Check sheet for the modelled part. Datum: model origin and axes. Units: mm. A direction names the side the tool comes from. Coordinates: 2 decimals unless noted, no trailing zeros. Loops run counter-clockwise (first coordinate to the right, second up) from the corner with the lowest first, then second, coordinate; pieces in that order, holes last. Notation, with made-up numbers: (-28, 8) - (-23, 8) arc R13 ccw to (-23, 32) - close; hole circle Ø1 at (-26, 46.25). An arc over 180 degrees is marked (long way). Use a Markdown table: item, result. Add a question column.
1) Draft check along X on faces 5 (the flat face through (5, 102, 12)), 6 (the flat face through (85, 100, 2)). Enter one of: pulls with the +X half, pulls with the -X half, needs draft (parallel to the pull), parting line crosses it, or undercut.
2) Sectioned sample at A-A, the plane x = 36. Enter the section's corners in (y, z).
3) Sectioned sample at D-D, the plane y = 64.5. Enter the section's corners in (x, z), then the cut area to 3 significant figures.
4) Go/stop test with flat-tipped pins: P1, Ø11, axis at x = 101, y = 93, coming from the +Z side; P2, Ø6, axis at x = 104, y = 77.5, coming from the +Z side; P3, Ø4, axis at y = 38, z = 13, coming from the -X side; P4, Ø1.4, axis at y = 67.5, z = 3, coming from the -X side. Record where each tip stops, or that it passes through.
5) Sectioned sample at B-B, the plane z = 51.5. Enter the section's corners in (x, y).
6) Thickness scan on line 1 (Y direction, x = 83, z = 3.3); line 2 (X direction, y = 100.5, z = 58); line 3 (Y direction, x = 16, z = 3). Record the ranges inside material, lowest first.
7) Sectioned sample at C-C, the plane y = 114. Enter the section's corners in (x, z), then the cut area to 3 significant figures.
8) Tool access check on faces 1 (the flat face through (5, 30, 12)), 2 (the flat face through (127, 12, 49.6)), 3 (the flat face through (142, 86, 41)), 4 (the flat face through (80, 55, 2)). Record the directions out of +Z, -Z, +X, -X, +Y, -Y that give a thin tool (end or side, any length) a straight path to the whole face; none if there is none.
from build123d import *

# Parameters (mm, degrees)
SKETCH_W            = 150
SKETCH_H            = 130
PAD_DEPTH           = 4.8
SKETCH001_R         = 3.3
POCKET_DEPTH        = 4.801
MIRROREDSKETCH_R    = 3.3
POCKET001_DEPTH     = 4.801
MIRROREDSKETCH001_R = 3.3
POCKET002_DEPTH     = 4.801
MIRROREDSKETCH002_R = 3.3
POCKET003_DEPTH     = 4.801
SKETCH002_W         = 2
SKETCH002_H         = 70
PAD001_DEPTH        = 5
SKETCH003_W         = 10
SKETCH003_H         = 2
PAD002_DEPTH        = 15
MIRROREDSKETCH003_W = 10
MIRROREDSKETCH003_H = 2
PAD003_DEPTH        = 15
PAD004_DEPTH        = 15
PAD005_DEPTH        = 15
PAD006_DEPTH        = 95
PAD007_DEPTH        = 95
SKETCH007_W         = 20
SKETCH007_H         = 60
POCKET004_DEPTH     = 5
PAD008_DEPTH        = 30
PAD009_DEPTH        = 30
SKETCH009_W         = 40
SKETCH009_H         = 70
POCKET005_DEPTH     = 4.801
SKETCH010_W         = 70
SKETCH010_H         = 20
POCKET006_DEPTH     = 4.801
POCKET007_DEPTH     = 4.801
POCKET008_DEPTH     = 4.801


with BuildPart() as part:
    # Sketch → Pad (new body)
    with BuildSketch(Plane.XY):
        with Locations((75, 65)):
            Rectangle(SKETCH_W, SKETCH_H)
    extrude(amount=PAD_DEPTH)

    # Sketch001 (on Face6 of Pad) → Pocket (cut, through all)
    with BuildSketch(Plane.XY.offset(4.8)):
        with Locations((16, 16)):
            Circle(SKETCH001_R)
    extrude(amount=-POCKET_DEPTH, mode=Mode.SUBTRACT)

    # MirroredSketch → Pocket001 (cut, through all)
    with BuildSketch(Plane.XY.offset(4.8)):
        with Locations((16, 114)):
            Circle(MIRROREDSKETCH_R)
    extrude(amount=-POCKET001_DEPTH, mode=Mode.SUBTRACT)

    # MirroredSketch001 → Pocket002 (cut, through all)
    with BuildSketch(Plane.XY.offset(4.8)):
        with Locations((83, 16)):
            Circle(MIRROREDSKETCH001_R)
    extrude(amount=-POCKET002_DEPTH, mode=Mode.SUBTRACT)

    # MirroredSketch002 → Pocket003 (cut, through all)
    with BuildSketch(Plane.XY.offset(4.8)):
        with Locations((83, 114)):
            Circle(MIRROREDSKETCH002_R)
    extrude(amount=-POCKET003_DEPTH, mode=Mode.SUBTRACT)

    # Sketch002 (on Face5 of Pocket003) → Pad001 (join)
    with BuildSketch(Plane.XY.offset(4.8)):
        with Locations((1, 65)):
            Rectangle(SKETCH002_W, SKETCH002_H)
    extrude(amount=PAD001_DEPTH)

    # Sketch003 (on Face5 of Pad001) → Pad002 (join)
    with BuildSketch(Plane.XY.offset(4.8)):
        with Locations((5, 29)):
            Rectangle(SKETCH003_W, SKETCH003_H)
    extrude(amount=PAD002_DEPTH)

    # MirroredSketch003 → Pad003 (join)
    with BuildSketch(Plane.XY.offset(4.8)):
        with Locations((5, 101)):
            Rectangle(MIRROREDSKETCH003_W, MIRROREDSKETCH003_H)
    extrude(amount=PAD003_DEPTH)

    # Sketch004 (on Face5 of Pad003) → Pad004 (join)
    with BuildSketch(Plane.XY.offset(4.8)):
        Polygon((96.4, 100), (96.4, 102), (106.4, 102), (106.4, 87), (104.4, 87), (104.4, 100), align=None)
    extrude(amount=PAD004_DEPTH)

    # Sketch005 (on Face5 of Pad004) → Pad005 (join)
    with BuildSketch(Plane.XY.offset(4.8)):
        Polygon((96.4, 30), (104.4, 30), (104.4, 43), (106.4, 43), (106.4, 28), (96.4, 28), align=None)
    extrude(amount=PAD005_DEPTH)

    # Sketch006 (on Face5 of Pad005) → Pad006 (join)
    with BuildSketch(Plane.XY.offset(4.8)):
        Polygon((109.8, 86), (109.8, 120.8), (145.8, 120.8), (145.8, 86), (141, 86), (141, 116), (114.6, 116), (114.6, 86), align=None)
    extrude(amount=PAD006_DEPTH)

    # MirroredSketch005 → Pad007 (join)
    with BuildSketch(Plane.XY.offset(4.8)):
        Polygon((145.8, 44), (145.8, 9.2), (109.8, 9.2), (109.8, 44), (114.6, 44), (114.6, 14), (141, 14), (141, 44), align=None)
    extrude(amount=PAD007_DEPTH)

    # Sketch007 (on Face33 of Pad007) → Pocket004 (cut)
    with BuildSketch(Plane.XZ.offset(-9.2)):
        with Locations((127.5, 79.6)):
            Rectangle(SKETCH007_W, SKETCH007_H)
    extrude(amount=-POCKET004_DEPTH, mode=Mode.SUBTRACT)

    # Sketch008 (on Face5 of Pocket004) → Pad008 (join)
    with BuildSketch(Plane.XY.offset(4.8)):
        Polygon((114.6, 86), (119.6, 86), (119.6, 111), (136, 111), (136, 86), (141, 86), (141, 116), (114.6, 116), align=None)
    extrude(amount=PAD008_DEPTH)

    # MirroredSketch006 → Pad009 (join)
    with BuildSketch(Plane.XY.offset(4.8)):
        Polygon((114.6, 44), (119.6, 44), (119.6, 19), (136, 19), (136, 44), (141, 44), (141, 14), (114.6, 14), align=None)
    extrude(amount=PAD009_DEPTH)

    # Sketch009 (on Face5 of Pad009) → Pocket005 (cut, through all)
    with BuildSketch(Plane.XY.offset(4.8)):
        with Locations((50, 65)):
            Rectangle(SKETCH009_W, SKETCH009_H)
    extrude(amount=-POCKET005_DEPTH, mode=Mode.SUBTRACT)

    # Sketch010 (on Face5 of Pocket005) → Pocket006 (cut, through all)
    with BuildSketch(Plane.XY.offset(4.8)):
        with Locations((55, 65)):
            Rectangle(SKETCH010_W, SKETCH010_H)
    extrude(amount=-POCKET006_DEPTH, mode=Mode.SUBTRACT)

    # Sketch011 (on Face5 of Pocket006) → Pocket007 (cut, through all)
    with BuildSketch(Plane.XY.offset(4.8)):
        with BuildLine():
            ThreePointArc((82.4, 30), (79.9, 27.5), (82.4, 25))
            Line((82.4, 25), (86.9, 25))
            ThreePointArc((86.9, 25), (89.4, 27.5), (86.9, 30))
            Line((82.4, 30), (86.9, 30))
        make_face()
    extrude(amount=-POCKET007_DEPTH, mode=Mode.SUBTRACT)

    # MirroredSketch007 → Pocket008 (cut, through all)
    with BuildSketch(Plane.XY.offset(4.8)):
        with BuildLine():
            ThreePointArc((82.4, 105), (79.9, 102.5), (82.4, 100))
            Line((82.4, 100), (86.9, 100))
            ThreePointArc((86.9, 100), (89.4, 102.5), (86.9, 105))
            Line((82.4, 105), (86.9, 105))
        make_face()
    extrude(amount=-POCKET008_DEPTH, mode=Mode.SUBTRACT)


solid = part.part
Solved:
| question | item | result |
|---|---|---|
| 1 | face 5 | needs draft |
| 1 | face 6 | undercut |
| 2 | outline | (0, 0) - (30, 0) - (30, 4.8) - (0, 4.8) - close; (100, 0) - (130, 0) - (130, 4.8) - (100, 4.8) - close |
| 3 | outline | (0, 0) - (20, 0) - (20, 4.8) - (2, 4.8) - (2, 9.8) - (0, 9.8) - close; (90, 0) - (150, 0) - (150, 4.8) - (90, 4.8) - close |
| 3 | area | 394 mm2 |
| 4 | P1 | stops at z = 19.8 |
| 4 | P2 | stops at z = 4.8 |
| 4 | P3 | stops at x = 104.4 |
| 4 | P4 | stops at x = 0 |
| 5 | outline | (109.8, 9.2) - (117.5, 9.2) - (117.5, 14) - (114.6, 14) - (114.6, 44) - (109.8, 44) - close; (109.8, 86) - (114.6, 86) - (114.6, 116) - (141, 116) - (141, 86) - (145.8, 86) - (145.8, 120.8) - (109.8, 120.8) - close; (137.5, 9.2) - (145.8, 9.2) - (145.8, 44) - (141, 44) - (141, 14) - (137.5, 14) - close |
| 6 | line 1 | y = 0 to 12.7, 19.3 to 25, 30 to 55, 75 to 100, 105 to 110.7, 117.3 to 130 |
| 6 | line 2 | x = 109.8 to 114.6, 141 to 145.8 |
| 6 | line 3 | y = 0 to 12.7, 19.3 to 110.7, 117.3 to 130 |
| 7 | outline | (0, 0) - (12.7, 0) - (12.7, 4.8) - (0, 4.8) - close; (19.3, 0) - (79.7, 0) - (79.7, 4.8) - (19.3, 4.8) - close; (86.3, 0) - (150, 0) - (150, 4.8) - (145.8, 4.8) - (145.8, 99.8) - (141, 99.8) - (141, 34.8) - (114.6, 34.8) - (114.6, 99.8) - (109.8, 99.8) - (109.8, 4.8) - (86.3, 4.8) - close |
| 7 | area | 2,360 mm2 |
| 8 | face 1 | +Z |
| 8 | face 2 | +Z, -Y |
| 8 | face 3 | +Z, +X |
| 8 | face 4 | +Z, -Z |
